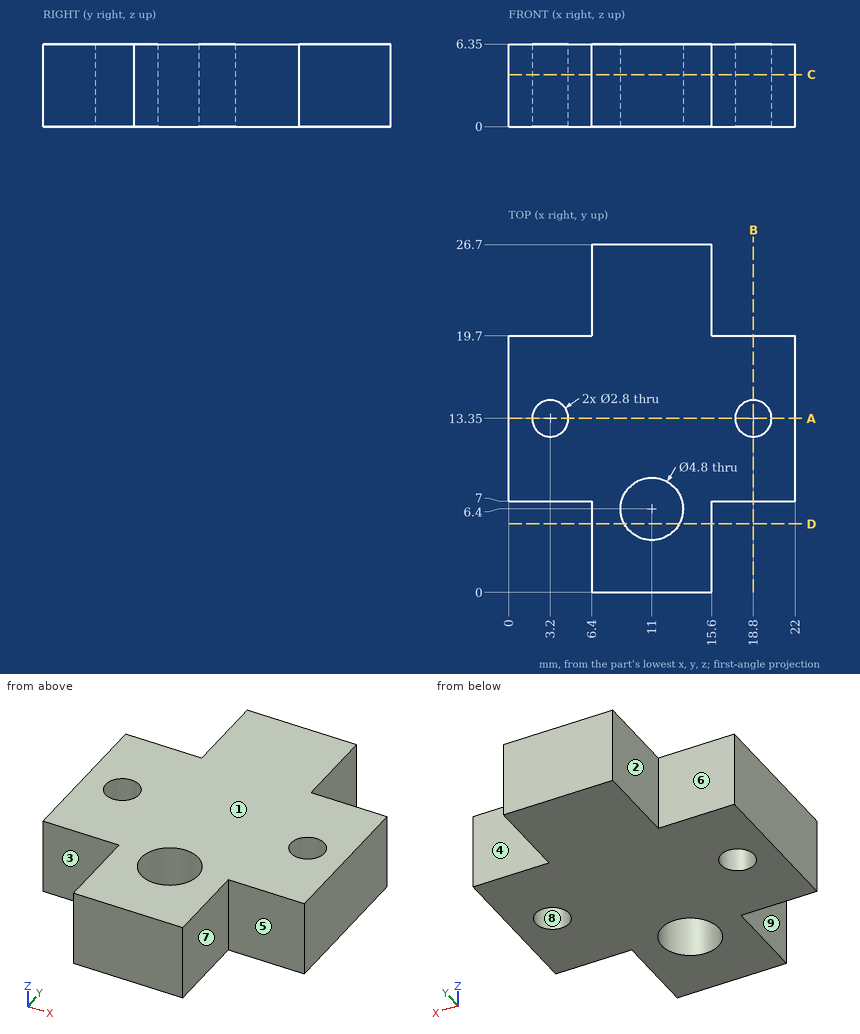
Answer from the drawing. Dimensions are ordinates in mm from the lowest x, y and z of the part. A direction names the side the tool comes from. Give positions to 0.01 mm unless a question says otherwise; leave off trailing zeros. Write each loop counter-clockwise with the first axis right and the second up, starting at its lowest first coordinate (ties: lowest second). Pieces come first, ordered by that corner, then holes. Notation, with made-up numbers: (88.25, 77.5) - (146.25, 77.5) arc R14 cw to (146.25, 99.5) - close; hole circle Ø8 at (-35, 44.25). An arc over 180 degrees is marked (long way). Answer in a Markdown table with one row per item. Add a question column.
Item 1: Determine the mould class of the marked faces 6, 7, 8 and 9 for opening direction X: pulls with the +X half, pulls with the -X half, needs draft (parallel to the pull), parting line crosses it, or undercut.
Item 2: Section A-A, the plane y = 13.35 is taken. Write down the section's boundary in (x, z), and give its area (3 significant figures).
Item 3: Section C-C, the plane z = 4 is taken. Write down the section's boundary in (x, y).
Item 4: Find the intervals of material crossed by L1, parallel to Y at x = 3.2, z = 2; L2, parallel to X at y = 24, z = 1.25; L3, parallel to Y at x = 21.25, z = 0.5, in increasing order.
Item 5: Section D-D, the plane y = 5.25 is taken. Write down the section's boundary in (x, z), and give its area (3 significant figures).
Item 6: Section B-B, the plane x = 18.8 is taken. Write down the section's boundary in (y, z).
Item 7: A tool of negligible diameter and unlimited length cuts with its end or side. For the marked faces 1, 2, 3, 4 and 5, from which of +Z, -Z, +X, -X, +Y, -Y can it reach the whole face along a straight path? Write none if from no direction.
Item 8: Flat-ended cylindrical pins translate along their axes: P1, Ø3, axis at y = 23.5, z = 3, coming from the +X side; P2, Ø2, axis at x = 3.2, y = 13.35, coming from the -Z side; P3, Ø1.9, axis at x = 18.5, z = 2.5, coming from the +Y side; P4, Ø1.9, axis at y = 2, z = 3.5, coming from the -X side. Find the tip coordinate at first contact, or state that the pin passes through.
Recorded:
| question | item | result |
|---|---|---|
| 1 | face 6 | needs draft |
| 1 | face 7 | pulls with the +X half |
| 1 | face 8 | undercut |
| 1 | face 9 | pulls with the -X half |
| 2 | outline | (0, 0) - (1.8, 0) - (1.8, 6.35) - (0, 6.35) - close; (4.6, 0) - (17.4, 0) - (17.4, 6.35) - (4.6, 6.35) - close; (20.2, 0) - (22, 0) - (22, 6.35) - (20.2, 6.35) - close |
| 2 | area | 104 mm2 |
| 3 | outline | (0, 7) - (6.4, 7) - (6.4, 0) - (15.6, 0) - (15.6, 7) - (22, 7) - (22, 19.7) - (15.6, 19.7) - (15.6, 26.7) - (6.4, 26.7) - (6.4, 19.7) - (0, 19.7) - close; hole circle Ø2.8 at (3.2, 13.35); hole circle Ø4.8 at (11, 6.4); hole circle Ø2.8 at (18.8, 13.35) |
| 4 | L1 | y = 7 to 11.95, 14.75 to 19.7 |
| 4 | L2 | x = 6.4 to 15.6 |
| 4 | L3 | y = 7 to 19.7 |
| 5 | outline | (6.4, 0) - (8.89, 0) - (8.89, 6.35) - (6.4, 6.35) - close; (13.11, 0) - (15.6, 0) - (15.6, 6.35) - (13.11, 6.35) - close |
| 5 | area | 31.7 mm2 |
| 6 | outline | (7, 0) - (11.95, 0) - (11.95, 6.35) - (7, 6.35) - close; (14.75, 0) - (19.7, 0) - (19.7, 6.35) - (14.75, 6.35) - close |
| 7 | face 1 | +Z, +X, -X, +Y, -Y |
| 7 | face 2 | +Z, -Z, -X, +Y |
| 7 | face 3 | +Z, -Z, -X, -Y |
| 7 | face 4 | +Z, -Z, +X, +Y |
| 7 | face 5 | +Z, -Z, +X, -Y |
| 8 | P1 | stops at x = 15.6 |
| 8 | P2 | passes through |
| 8 | P3 | stops at y = 19.7 |
| 8 | P4 | stops at x = 6.4 |
